Source: CAD feature listing. Evaluate the final solid. Frame: model axes, mm. Coordinates: 2 decimals unless noted, no trailing zeros. Order: outer loops, then holes, each group sorted by start corner. A loop starts at its lowest first (then second) coordinate and runs counter-clockwise, first axis right, second up.
```python
from build123d import *

# Parameters (mm, degrees)
F1_R     = 7.5
F1_W     = 20
F1_H     = 15
F1_H_2   = 5
F2_DEPTH = 5


with BuildPart() as f2:
    # F1 (on Right) → F2 (new body)
    with BuildSketch(Plane.YZ):
        Polygon((0, 60), (0, 0), (2.5, 0), (22.5, 0), (42.5, 0), (62.5, 0), (272.5, 0), (292.5, 0), (312.5, 0), (332.5, 0), (335, 0), (335, 60), (332.5, 60), (312.5, 60), (292.5, 60), (272.5, 60), (62.5, 60), (42.5, 60), (22.5, 60), (2.5, 60), align=None)
        with Locations((22.5, 20)):
            Circle(F1_R, mode=Mode.SUBTRACT)
        Polygon((247.5, 10), (237.5, 10), (247.5, 20), align=None, mode=Mode.SUBTRACT)
        Polygon((97.5, 10), (87.5, 10), (127.5, 50), (137.5, 50), align=None, mode=Mode.SUBTRACT)
        Polygon((122.5, 10), (112.5, 10), (152.5, 50), (162.5, 50), align=None, mode=Mode.SUBTRACT)
        Polygon((147.5, 10), (137.5, 10), (177.5, 50), (187.5, 50), align=None, mode=Mode.SUBTRACT)
        Polygon((102.5, 50), (112.5, 50), (87.5, 25), (87.5, 35), align=None, mode=Mode.SUBTRACT)
        Polygon((172.5, 10), (162.5, 10), (202.5, 50), (212.5, 50), align=None, mode=Mode.SUBTRACT)
        Polygon((222.5, 10), (212.5, 10), (247.5, 45), (247.5, 35), align=None, mode=Mode.SUBTRACT)
        Polygon((197.5, 10), (187.5, 10), (227.5, 50), (237.5, 50), align=None, mode=Mode.SUBTRACT)
        with BuildLine():
            Line((312.5, 32.5), (272.5, 32.5))
            ThreePointArc((272.5, 32.5), (265, 40), (272.5, 47.5))
            Line((272.5, 47.5), (312.5, 47.5))
            ThreePointArc((312.5, 47.5), (320, 40), (312.5, 32.5))
        make_face(mode=Mode.SUBTRACT)
        with Locations((12.5, -7.5)):
            Rectangle(F1_W, F1_H)
        with Locations((12.5, 62.5)):
            Rectangle(F1_W, F1_H_2)
        with Locations((52.5, -2.5)):
            Rectangle(F1_W, F1_H_2)
        with Locations((52.5, 62.5)):
            Rectangle(F1_W, F1_H_2)
        with Locations((282.5, -2.5)):
            Rectangle(F1_W, F1_H_2)
        with Locations((282.5, 62.5)):
            Rectangle(F1_W, F1_H_2)
        with Locations((322.5, -7.5)):
            Rectangle(F1_W, F1_H)
        with Locations((322.5, 62.5)):
            Rectangle(F1_W, F1_H_2)
    extrude(amount=F2_DEPTH)


solid = f2.part
```
1. Section query A-A, the plane y = 119. Output: boundary loops of the cut face in (x, z), plus the area to 4 significant figures.
2. Material intervals for line 1 along Y through (x, z) = (1.95, -7); line 2 along Z through (x, y) = (3.4, 157); line 3 along Z through (x, y) = (1.1, 289), sorted ascending.
3. Contact query for flat-ended pins moving along their axis: P1, Ø1.5, axis at x = 2.5, y = 244.5, coming from the +Z side; P2, Ø2.5, axis at x = 2.5, y = 285.5, coming from the -Z side; P3, Ø2, axis at y = 208, z = 34, coming from the -X side; P4, Ø0.8, axis at x = 3, y = 1.5, coming from the -Z side. Output: stop coordinate, or through.
4. Section query B-B, the plane y = 26.5. Output: boundary loops of the cut face in (x, z).
5. Section query C-C, the plane z = 40. Count the separate pieces of the cut face and the enclosed holes in it, plus the area to 4 significant figures.
6. Draft query along Y for faces 1 (the flat face through (5, 165, 26)), 2 (the flat face through (2.5, 132.2, 29.7)). Return one class per face: +Y half, -Y half, draft (parallel to the pull), parting line (faces both ways), or undercut.
Answer key:
1. outline: (0, 0) - (5, 0) - (5, 10) - (0, 10) - close; (0, 16.5) - (5, 16.5) - (5, 31.5) - (0, 31.5) - close; (0, 41.5) - (5, 41.5) - (5, 60) - (0, 60) - close
1. area: 217.5 mm2
2. line 1: y = 2.5 to 22.5, 312.5 to 332.5
2. line 2: z = 0 to 19.5, 29.5 to 44.5, 50 to 60
2. line 3: z = -5 to 32.5, 47.5 to 65
3. P1: stops at z = 60
3. P2: stops at z = -5
3. P3: stops at x = 0
3. P4: stops at z = 0
4. outline: (0, 0) - (5, 0) - (5, 13.66) - (0, 13.66) - close; (0, 26.34) - (5, 26.34) - (5, 60) - (0, 60) - close
5. separate pieces: 9
5. enclosed holes: 0
5. area: 1,075 mm2
6. face 1: draft
6. face 2: undercut
